Here's how the part is built. I have some questions about the finished solid (model axes, mm). A direction names the side the tool comes from. Give positions to 0.01 mm unless a question says otherwise; leave off trailing zeros. Order: outer loops, then holes, each group sorted by start corner. A loop starts at its lowest first (then second) coordinate and runs counter-clockwise, first axis right, second up. Notation, with made-up numbers: (-23.75, 51) -> (-15.75, 51) arc R12 ccw to (-15.75, 62) -> close; hole circle Ø5 at (50, -32.75). An arc over 180 degrees is marked (long way). Write each question's results on one line, items separated by ' | '. Start each with the question number.
Q1. For faces 4 (the face through (-61.505, -6, 183)), 5 (the face through (-137.705, -6, -97)), 6 (the face through (173, -6, 36.809)), 7 (the face through (-131, -6, -90.191)), which set-ups out of +Z, -Z, +X, -X, +Y, -Y let a thin tool reach every point of the face, with its end or its side?
Q2. Imagine slicing it at B-B, the plane x = 122. Please give me the cut outline in (y, z), then the cut area to 3 significant figures.
Q3. Imagine slicing it at A-A, the plane z = 18.5. Please give me the cut outline in (x, y), then the cut area to 3 significant figures.
Q4. I need wall thicknesses on line 1 along Z through (x, y) = (19, -12); line 2 along X through (y, z) = (-2.25, 116). Which ranges of each line are inside material? Lowest first, please. Write a range as [from, to].
Q5. I'm going to push flat-ended pins straight in: pin 1 (4 mm diameter, centred on y = -9.5, z = -60.5, fed in from +X); pin 2 (6.5 mm diameter, centred on x = -80, y = -8.5, fed in from +Z). Where does each tip first touch, or does it pass through?
Q6. Thinking about a two-plate mould opening in X: for faces 1 (the face through (-137.705, -6, 81)), 2 (the face through (173, -6, 138.409)), 3 (the face through (65.495, -6, 183)), which applies, pulls with the +X half, pulls with the -X half, needs draft (parallel to the pull), parting line crosses it, or undercut?
```python
from build123d import *

# Parameters (mm, degrees)
F0_W     = 12.7
F0_H     = 12.7
F1_DEPTH = 12.7


with BuildPart() as f1:
    # F0 (on Front) → F1 (new body)
    with BuildSketch(Plane.XZ):
        with Locations((-131.354641, 182.858769)):
            Rectangle(F0_W, F0_H)
        with Locations((-131.354641, 157.458769)):
            Rectangle(F0_W, F0_H)
        Polygon((-112.304641, 189.208769), (-125.004641, 189.208769), (-125.004641, 176.508769), (-125.004641, 163.808769), (-125.004641, 151.108769), (-125.004641, 138.408769), (-125.004641, 125.708769), (-125.004641, 113.008769), (-125.004641, 100.308769), (-125.004641, 87.608769), (-125.004641, 74.908769), (-125.004641, 62.208769), (-125.004641, 49.508769), (-125.004641, 36.808769), (-125.004641, 24.108769), (-125.004641, 11.408769), (-125.004641, -1.291231), (-125.004641, -13.991231), (-125.004641, -26.691231), (-125.004641, -39.391231), (-125.004641, -52.091231), (-125.004641, -64.791231), (-125.004641, -77.491231), (-125.004641, -90.191231), (-125.004641, -102.891231), (167.095359, -102.891231), (167.095359, -90.191231), (167.095359, -77.491231), (167.095359, -64.791231), (167.095359, -52.091231), (167.095359, -39.391231), (167.095359, -26.691231), (167.095359, -13.991231), (167.095359, -1.291231), (167.095359, 11.408769), (167.095359, 24.108769), (167.095359, 36.808769), (167.095359, 49.508769), (167.095359, 62.208769), (167.095359, 74.908769), (167.095359, 87.608769), (167.095359, 100.308769), (167.095359, 113.008769), (167.095359, 125.708769), (167.095359, 138.408769), (167.095359, 151.108769), (167.095359, 163.808769), (167.095359, 176.508769), (167.095359, 189.208769), (154.395359, 189.208769), (154.395359, 176.508769), (141.695359, 176.508769), (141.695359, 189.208769), (128.995359, 189.208769), (128.995359, 176.508769), (116.295359, 176.508769), (116.295359, 189.208769), (103.595359, 189.208769), (103.595359, 176.508769), (90.895359, 176.508769), (90.895359, 189.208769), (78.195359, 189.208769), (78.195359, 176.508769), (65.495359, 176.508769), (65.495359, 189.208769), (52.795359, 189.208769), (52.795359, 176.508769), (40.095359, 176.508769), (40.095359, 189.208769), (27.395359, 189.208769), (27.395359, 176.508769), (14.695359, 176.508769), (14.695359, 189.208769), (1.995359, 189.208769), (1.995359, 176.508769), (-10.704641, 176.508769), (-10.704641, 189.208769), (-23.404641, 189.208769), (-23.404641, 176.508769), (-36.104641, 176.508769), (-36.104641, 189.208769), (-48.804641, 189.208769), (-48.804641, 176.508769), (-61.504641, 176.508769), (-61.504641, 189.208769), (-74.204641, 189.208769), (-74.204641, 176.508769), (-86.904641, 176.508769), (-86.904641, 189.208769), (-99.604641, 189.208769), (-99.604641, 176.508769), (-112.304641, 176.508769), align=None)
        with Locations((173.445359, 182.858769)):
            Rectangle(F0_W, F0_H)
        with Locations((173.445359, 157.458769)):
            Rectangle(F0_W, F0_H)
        with Locations((173.445359, 132.058769)):
            Rectangle(F0_W, F0_H)
        with Locations((173.445359, 106.658769)):
            Rectangle(F0_W, F0_H)
        with Locations((173.445359, 81.258769)):
            Rectangle(F0_W, F0_H)
        with Locations((173.445359, 55.858769)):
            Rectangle(F0_W, F0_H)
        with Locations((173.445359, 30.458769)):
            Rectangle(F0_W, F0_H)
        with Locations((173.445359, 5.058769)):
            Rectangle(F0_W, F0_H)
        with Locations((173.445359, -20.341231)):
            Rectangle(F0_W, F0_H)
        with Locations((173.445359, -45.741231)):
            Rectangle(F0_W, F0_H)
        with Locations((173.445359, -71.141231)):
            Rectangle(F0_W, F0_H)
        with Locations((173.445359, -96.541231)):
            Rectangle(F0_W, F0_H)
        with Locations((-131.354641, -96.541231)):
            Rectangle(F0_W, F0_H)
        with Locations((-131.354641, -71.141231)):
            Rectangle(F0_W, F0_H)
        with Locations((-131.354641, -45.741231)):
            Rectangle(F0_W, F0_H)
        with Locations((-131.354641, -20.341231)):
            Rectangle(F0_W, F0_H)
        with Locations((-131.354641, 5.058769)):
            Rectangle(F0_W, F0_H)
        with Locations((-131.354641, 30.458769)):
            Rectangle(F0_W, F0_H)
        with Locations((-131.354641, 55.858769)):
            Rectangle(F0_W, F0_H)
        with Locations((-131.354641, 81.258769)):
            Rectangle(F0_W, F0_H)
        with Locations((-131.354641, 106.658769)):
            Rectangle(F0_W, F0_H)
        with Locations((-131.354641, 132.058769)):
            Rectangle(F0_W, F0_H)
    extrude(amount=F1_DEPTH)


with BuildPart() as f2_1:
    # F2: copy of F1
    add(f1.part)


solid = f2_1.part
```
Geometry check:
1) face 4: +Z, +Y, -Y | face 5: +Z, -Z, -X, +Y, -Y | face 6: +X, +Y, -Y | face 7: -X, +Y, -Y
2) outline: (-12.7, -102.89) -> (0, -102.89) -> (0, 176.51) -> (-12.7, 176.51) -> close | area: 3,550 mm²
3) outline: (-125, -12.7) -> (167.1, -12.7) -> (167.1, 0) -> (-125, 0) -> close | area: 3,710 mm²
4) line 1: [-102.89, 176.51] | line 2: [-125, 167.1]
5) pin 1: x = 167.1 | pin 2: z = 176.51
6) face 1: pulls with the -X half | face 2: needs draft | face 3: undercut
